Autodesk Inventor part; units mm, degrees
ref_plane "YZ Plane" through (0, 0, 0) normal (1, 0, 0) x (0, 1, 0)
ref_plane "XZ Plane" through (0, 0, 0) normal (0, 1, 0) x (-1, 0, 0)
ref_plane "XY Plane" through (0, 0, 0) normal (0, 0, 1) x (1, 0, 0)
ref_plane "Work Plane1" through (-10.7838, -0.756, 0) normal (0, 0, 1) x (1, 0, 0)
sketch "Sketch1" plane through (-10.7838, -0.756, 0) normal (0, 0, 1) x (1, 0, 0)
  line L0 (-33.2162, 0.756) -> (-33.2162, 6.756)
  line L1 (-33.2162, 0.756) -> (-23.2162, 0.756)
  line L2 (-23.2162, 0.756) -> (-23.2162, 6.756)
  line L3 (-23.2162, 6.756) -> (-33.2162, 6.756)
  line L4 (-3.2162, 0.756) -> (-3.2162, 6.756)
  line L5 (-3.2162, 6.756) -> (-13.2162, 6.756)
  line L6 (-13.2162, 0.756) -> (-13.2162, 6.756)
  line L7 (-13.2162, 0.756) -> (-3.2162, 0.756)
  line L8 (-135.7005, 28.256) -> (83.2995, 28.256)
  line L9 (83.2995, 43.256) -> (-135.7005, 43.256)
  line L10 (-43.2162, 0.756) -> (-43.2162, 6.756)
  line L11 (-43.2162, 6.756) -> (-47.2162, 6.756)
  line L12 (-47.2162, 0.756) -> (-47.2162, 6.756)
  line L13 (-47.2162, 0.756) -> (-43.2162, 0.756)
  line L14 (16.7838, 6.756) -> (10.7838, 6.756)
  line L15 (10.7838, 0.756) -> (10.7838, 6.756)
  line L16 (10.7838, 0.756) -> (16.7838, 0.756)
  line L17 (16.7838, 0.756) -> (16.7838, 6.756)
  line L18 (-53.2162, 6.756) -> (-53.2162, 0.756)
  line L19 (-47.2162, 0.756) -> (-53.2162, 0.756)
  line L20 (-47.2162, 0.756) -> (-47.2162, 6.756)
  line L21 (-47.2162, 6.756) -> (-53.2162, 6.756)
  line L22 (-53.2162, 6.756) -> (16.7838, 6.756)
  line L23 (16.7838, 6.756) -> (16.7838, 28.256)
  line L24 (16.7838, 28.256) -> (-53.2162, 28.256)
  line L25 (-53.2162, 28.256) -> (-53.2162, 6.756)
  line L26 (-53.2162, 12.506) -> (-47.2162, 12.506)
  line L27 (-47.2162, 12.506) -> (-47.2162, 22.506)
  line L28 (-47.2162, 22.506) -> (-53.2162, 22.506)
  line L29 (-53.2162, 22.506) -> (-53.2162, 12.506)
  line L30 (16.7838, 22.506) -> (10.7838, 22.506)
  line L31 (10.7838, 22.506) -> (10.7838, 12.506)
  line L32 (10.7838, 12.506) -> (16.7838, 12.506)
  line L33 (16.7838, 12.506) -> (16.7838, 22.506)
  line L34 (-38.2162, 28.256) -> (-28.2162, 28.256)
  line L35 (-28.2162, 28.256) -> (-28.2162, 22.256)
  line L36 (-28.2162, 22.256) -> (-38.2162, 22.256)
  line L37 (-38.2162, 22.256) -> (-38.2162, 28.256)
  line L38 (1.7838, 28.256) -> (-8.2162, 28.256)
  line L39 (-8.2162, 28.256) -> (-8.2162, 22.256)
  line L40 (-8.2162, 22.256) -> (1.7838, 22.256)
  line L41 (1.7838, 22.256) -> (1.7838, 28.256)
  point P0 (-47.2162, 17.506)
  point P1 (-53.2162, 17.506)
  point P2 (10.7838, 17.506)
  point P3 (16.7838, 17.506)
extrude "Plate1" add sketch "Sketch1" along normal blind 6 contours L0 L3 L2 L1 | L22 L11 L21 L25 L26 L27 L28 L8 L37 L36 L35 L39 L40 L41 L23 L30 L31 L32 L14 L5 L3 | L10 L13 L12 L11 | L5 L4 L7 L6 | L12 L19 L18 L21 | L14 L17 L16 L15
equation "\"d10\" = Thickness"
equation "\"BendRadius\" = Thickness"
equation "\"BendReliefWidth\" = Thickness"
equation "\"BendReliefDepth\" = 0.5 * Thickness"
equation "\"CornerReliefSize\" = 4 * Thickness"
equation "\"MinimumRemnant\" = 2 * Thickness"
equation "\"TransitionRadius\" = BendRadius"
equation "\"JacobiRadiusSize\" = BendRadius"
equation "\"GapSize\" = Thickness"
equation "\"d9\" = d8"
properties part number "onderzijde joystickdoosje" material "Wood (Birch)"
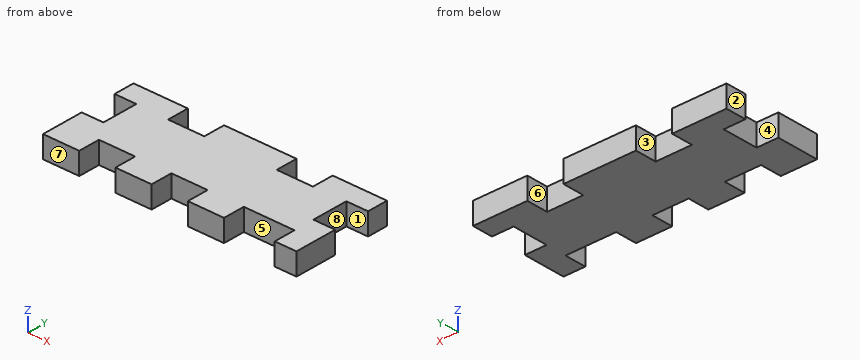
Geometry: final body of the model. Coordinates: model frame, mm. Face numbers are marked on the shaded views. A direction names the side the tool comes from. Coordinates: 2 decimals unless noted, no trailing zeros. Loops run counter-clockwise (first coordinate to the right, second up) from the corner with the lowest first, then second, coordinate; pieces in that order, holes last. Notation, with made-up numbers: (65.5, -23) - (118.5, -23) arc R30 ccw to (118.5, 5) - close; hole circle Ø7 at (57, 55.5). An arc over 180 degrees is marked (long way). Put each result on its own line as item: value. Start each with the question number.
Q1. Cut plane D-D, the plane y = 17. Return loops of the section in (x, z).
Q2. Pull-direction query (Y, two-part tool) for the marked faces 6, 7 and 8; classes: released by +Y, released by -Y, zero draft, split by the parting line, or undercut.
Q3. Pin query (flat end, axial travel): pin 1 Ø3 at (y, z) = (17, 3.5) entering from -X; pin 2 Ø1.8 at (y, z) = (16, 3.5) entering from +X. Return the tip coordinate at first contact, or that it passes through.
Q4. Line query: line 1 (X direction, y = 25.5, z = 5.4); line 2 (X direction, y = 5.25, z = 3.7); line 3 (X direction, y = 20.5, z = 3.8). Output: solid intervals per line, ascending.
Q5. Cut plane C-C, the plane x = -17. Return loops of the section in (y, z), and give its area (3 significant figures).
Q6. Set-up query: the marked faces 1, 2, 3, 4 and 5. Return all of +Z, -Z, +X, -X, +Y, -Y with unobstructed straight access to the full face (end or side cutting, diameter ignored); none if empty.
Q7. Cut plane A-A, the plane y = 3.25. Return loops of the section in (x, z), and give its area (3 significant figures).
Filled sheet:
1. outline: (-58, 0) - (0, 0) - (0, 6) - (-58, 6) - close
2. face 6: zero draft
2. face 7: released by -Y
2. face 8: undercut
3. pin 1: x = -58
3. pin 2: x = 0
4. line 1: -64 to -49, -39 to -19, -9 to 6
4. line 2: -64 to -54, -44 to -34, -24 to -14, 0 to 6
4. line 3: -58 to 0
5. outline: (0, 0) - (21.5, 0) - (21.5, 6) - (0, 6) - close
5. area: 129 mm²
6. face 1: +Z, -Z, +X
6. face 2: +Z, -Z, -X, +Y, -Y
6. face 3: +Z, -Z, +Y
6. face 4: +Z, -Z, -X
6. face 5: +Z, -Z, -Y
7. outline: (-64, 0) - (-54, 0) - (-54, 6) - (-64, 6) - close; (-44, 0) - (-34, 0) - (-34, 6) - (-44, 6) - close; (-24, 0) - (-14, 0) - (-14, 6) - (-24, 6) - close; (0, 0) - (6, 0) - (6, 6) - (0, 6) - close
7. area: 216 mm²
